from build123d import *

# Parameters (mm, degrees)
F0_W     = 25
F0_H     = 25
F0_R     = 2.5
F0_W_2   = 13
F0_H_2   = 13
F1_DEPTH = 1.2
F0_R_2   = 0.9
F2_DEPTH = 7.5
F3_R     = 2.655635


with BuildPart() as f1:
    # F0 (on Top) → F1 (new body)
    with BuildSketch(Plane.XY):
        Rectangle(F0_W, F0_H)
        with Locations((-8.7, -8.7)):
            Circle(F0_R, mode=Mode.SUBTRACT)
        with Locations((8.7, -8.7)):
            Circle(F0_R, mode=Mode.SUBTRACT)
        with Locations((-8.7, 8.7)):
            Circle(F0_R, mode=Mode.SUBTRACT)
        Rectangle(F0_W_2, F0_H_2, mode=Mode.SUBTRACT)
        with Locations((8.7, 8.7)):
            Circle(F0_R, mode=Mode.SUBTRACT)
    extrude(amount=F1_DEPTH)

    # F0 (on Top) → F2 (join)
    with BuildSketch(Plane.XY):
        with Locations((-8.7, 8.7)):
            Circle(F0_R)
        with Locations((-8.7, 8.7)):
            Circle(F0_R_2, mode=Mode.SUBTRACT)
        with Locations((8.7, 8.7)):
            Circle(F0_R)
        with Locations((8.7, 8.7)):
            Circle(F0_R_2, mode=Mode.SUBTRACT)
        with Locations((-8.7, -8.7)):
            Circle(F0_R)
        with Locations((-8.7, -8.7)):
            Circle(F0_R_2, mode=Mode.SUBTRACT)
        with Locations((8.7, -8.7)):
            Circle(F0_R)
        with Locations((8.7, -8.7)):
            Circle(F0_R_2, mode=Mode.SUBTRACT)
    extrude(amount=F2_DEPTH)

    # F3
    f3_edges = [f1.edges().sort_by_distance(p)[0] for p in [
        (12.5, -12.5, 0.6),
        (12.5, 12.5, 0.6),
        (-12.5, 12.5, 0.6),
        (-12.5, -12.5, 0.6),
        (-6.5, 6.5, 0.6),
        (-6.5, -6.5, 0.6),
        (6.5, -6.5, 0.6),
        (6.5, 6.5, 0.6),
    ]]
    fillet(f3_edges, radius=F3_R)


solid = f1.part
Could you check a few things on this model? Use its own coordinates, in mm. A direction names the side the tool comes from. Give positions to 0.01 mm unless a question says otherwise; leave off trailing zeros. Order: outer loops, then holes, each group sorted by start corner. A loop starts at its lowest first (then second) coordinate and runs counter-clockwise, first axis right, second up.
1. Thinking about a two-plate mould opening in X: for faces 1 (the flat face through (10, -9, 7.5)), 2 (the cylindrical face through (-11.743, -11.701, 0.608)), 3 (the cylindrical face through (7.99, -9.25, 3.7)), which applies, +X half, -X half, draft (parallel to the pull), parting line (faces both ways), or undercut?
Answers below:
face 1: draft
face 2: -X half
face 3: undercut
2. Suppose I cut it at B-B (y = -8.7). Write out the boundary of the cut face in (x, z), plus the area to 3 significant figures.
Answers below:
outline: (-12.5, 0) - (-9.6, 0) - (-9.6, 7.5) - (-11.2, 7.5) - (-11.2, 1.2) - (-12.5, 1.2) - close; (-7.8, 0) - (7.8, 0) - (7.8, 7.5) - (6.2, 7.5) - (6.2, 1.2) - (-6.2, 1.2) - (-6.2, 7.5) - (-7.8, 7.5) - close; (9.6, 0) - (12.5, 0) - (12.5, 1.2) - (11.2, 1.2) - (11.2, 7.5) - (9.6, 7.5) - close
area: 66.0 mm2
3. Suppose I cut it at A-A (z = 4.5). Write out the boundary of the cut face in (x, y), plus the area to 3 significant figures.
Answers below:
outline: circle Ø5 at (-8.7, -8.7); circle Ø5 at (-8.7, 8.7); circle Ø5 at (8.7, -8.7); circle Ø5 at (8.7, 8.7); hole circle Ø1.8 at (-8.7, -8.7); hole circle Ø1.8 at (-8.7, 8.7); hole circle Ø1.8 at (8.7, -8.7); hole circle Ø1.8 at (8.7, 8.7)
area: 68.4 mm2
4. For pin 1 (4 mm diameter, centred on x = -3.5, y = -6, fed in from +Z), with a flat end and sliding along its axis, tell me the tip position at first contact or that it passes through.
Answers below:
pin 1: stops at z = 1.2
5. I need wall thicknesses on L1, parallel to Y at x = 8.7, z = 5; L2, parallel to Y at x = 5.25, z = 0.5; L3, parallel to Z at x = -9.25, y = 5.5. Which ranges of each line are inside material? Lowest first, please.
Answers below:
L1: y = -11.2 to -9.6, -7.8 to -6.2, 6.2 to 7.8, 9.6 to 11.2
L2: y = -12.5 to -6.1, 6.1 to 12.5
L3: z = 0 to 1.2
6. Suppose I cut it at D-D (x = 1.5). Write out the boundary of the cut face in (y, z).
Answers below:
outline: (-12.5, 0) - (-6.5, 0) - (-6.5, 1.2) - (-12.5, 1.2) - close; (6.5, 0) - (12.5, 0) - (12.5, 1.2) - (6.5, 1.2) - close
7. Which directions (+Z, -Z, +X, -X, +Y, -Y) give clear straight access to the entire face, cutting with the end or side of a thin tool? Please do faces 4 (the cylindrical face through (-5.701, -5.743, 0.608)), 5 (the flat face through (10, 9, 7.5)), 6 (the cylindrical face through (-9.03, -6.22, 4.31)).
Answers below:
face 4: +Z, -Z
face 5: +Z, +X, -X, +Y, -Y
face 6: +Z
